from build123d import *

# Parameters (mm, degrees)
SKETCH_1_R         = 3.4
EXTRUDE_1267_DEPTH = 150


with BuildPart() as part:
    # 草圖1 → Extrude 1267 (new body, symmetric)
    with BuildSketch(Plane.XY):
        with BuildLine():
            Line((4.3, 25), (25, 25))
            Line((25, 25), (25, 4.3))
            Line((25, 4.3), (22, 4.3))
            Line((22, 4.3), (22, 6.687301399))
            Line((22, 6.687301399), (14.5, 6.687301399))
            ThreePointArc((14.5, 6.687301399), (10.2, 0), (14.5, -6.687301399))
            Line((14.5, -6.687301399), (22, -6.687301399))
            Line((22, -6.687301399), (22, -4.3))
            Line((22, -4.3), (25, -4.3))
            Line((25, -4.3), (25, -25))
            Line((25, -25), (4.3, -25))
            Line((4.3, -25), (4.3, -22))
            Line((4.3, -22), (6.687301399, -22))
            Line((6.687301399, -22), (6.687301399, -14.5))
            ThreePointArc((6.687301399, -14.5), (0, -10.2), (-6.687301399, -14.5))
            Line((-6.687301399, -14.5), (-6.687301399, -22))
            Line((-6.687301399, -22), (-4.3, -22))
            Line((-4.3, -22), (-4.3, -25))
            Line((-4.3, -25), (-25, -25))
            Line((-25, -25), (-25, -4.3))
            Line((-25, -4.3), (-22, -4.3))
            Line((-22, -4.3), (-22, -6.687301399))
            Line((-22, -6.687301399), (-14.5, -6.687301399))
            ThreePointArc((-14.5, -6.687301399), (-10.2, 0), (-14.5, 6.687301399))
            Line((-14.5, 6.687301399), (-22, 6.687301399))
            Line((-22, 6.687301399), (-22, 4.3))
            Line((-22, 4.3), (-25, 4.3))
            Line((-25, 4.3), (-25, 25))
            Line((-25, 25), (-4.3, 25))
            Line((-4.3, 25), (-4.3, 22))
            Line((-4.3, 22), (-6.687301399, 22))
            Line((-6.687301399, 22), (-6.687301399, 14.5))
            ThreePointArc((-6.687301399, 14.5), (0, 10.2), (6.687301399, 14.5))
            Line((6.687301399, 14.5), (6.687301399, 22))
            Line((6.687301399, 22), (4.3, 22))
            Line((4.3, 22), (4.3, 25))
        make_face()
        with Locations((12.75, 12.75)):
            Circle(SKETCH_1_R, mode=Mode.SUBTRACT)
        with Locations((12.75, -12.75)):
            Circle(SKETCH_1_R, mode=Mode.SUBTRACT)
        with Locations((-12.75, -12.75)):
            Circle(SKETCH_1_R, mode=Mode.SUBTRACT)
        with Locations((-12.75, 12.75)):
            Circle(SKETCH_1_R, mode=Mode.SUBTRACT)
        with BuildLine():
            Line((9.35, 23), (23, 23))
            Line((23, 23), (23, 9.35))
            Line((23, 9.35), (16.945235393, 9.35))
            ThreePointArc((16.945235393, 9.35), (16.568376618, 16.568376618), (9.35, 16.945235393))
            Line((9.35, 16.945235393), (9.35, 23))
        make_face(mode=Mode.SUBTRACT)
        with BuildLine():
            Line((9.35, -23), (9.35, -16.945235393))
            ThreePointArc((9.35, -16.945235393), (16.568376618, -16.568376618), (16.945235393, -9.35))
            Line((16.945235393, -9.35), (23, -9.35))
            Line((23, -9.35), (23, -23))
            Line((23, -23), (9.35, -23))
        make_face(mode=Mode.SUBTRACT)
        with BuildLine():
            Line((-9.35, -23), (-23, -23))
            Line((-23, -23), (-23, -9.35))
            Line((-23, -9.35), (-16.945235393, -9.35))
            ThreePointArc((-16.945235393, -9.35), (-16.568376618, -16.568376618), (-9.35, -16.945235393))
            Line((-9.35, -16.945235393), (-9.35, -23))
        make_face(mode=Mode.SUBTRACT)
        with BuildLine():
            Line((-9.35, 23), (-9.35, 16.945235393))
            ThreePointArc((-9.35, 16.945235393), (-16.568376618, 16.568376618), (-16.945235393, 9.35))
            Line((-16.945235393, 9.35), (-23, 9.35))
            Line((-23, 9.35), (-23, 23))
            Line((-23, 23), (-9.35, 23))
        make_face(mode=Mode.SUBTRACT)
        with BuildLine():
            ThreePointArc((11.864845961, 7.423040048), (8.2, 0), (11.864845961, -7.423040048))
            ThreePointArc((11.864845961, -7.423040048), (8.931623382, -8.931623382), (7.423040048, -11.864845961))
            ThreePointArc((7.423040048, -11.864845961), (0, -8.2), (-7.423040048, -11.864845961))
            ThreePointArc((-7.423040048, -11.864845961), (-8.931623382, -8.931623382), (-11.864845961, -7.423040048))
            ThreePointArc((-11.864845961, -7.423040048), (-8.2, 0), (-11.864845961, 7.423040048))
            ThreePointArc((-11.864845961, 7.423040048), (-8.931623382, 8.931623382), (-7.423040048, 11.864845961))
            ThreePointArc((-7.423040048, 11.864845961), (0, 8.2), (7.423040048, 11.864845961))
            ThreePointArc((7.423040048, 11.864845961), (8.931623382, 8.931623382), (11.864845961, 7.423040048))
        make_face(mode=Mode.SUBTRACT)
    extrude(amount=EXTRUDE_1267_DEPTH, both=True)


solid = part.part
Work out the finished part from the listing and answer in its coordinate system (mm). A direction names the side the tool comes from. Coordinates: 2 decimals unless noted, no trailing zeros. Order: outer loops, then holes, each group sorted by start corner. A loop starts at its lowest first (then second) coordinate and runs counter-clockwise, first axis right, second up. Notation, with made-up numbers: (-7.75, 21) - (29.25, 21) arc R15 ccw to (29.25, 46) - close; hole circle Ø4 at (80, 18.25). An arc over 180 degrees is marked (long way). Put each result on its own line as item: value. Start each with the question number.
1) Find section A-A (x = -0.5). Give the vertices of the cut face in (y, z), plus the area to 3 significant figures.
2) For a pull along Y with two mould halves and no side action, classify faces 3 (the flat face through (15, 25, 2)), 4 (the flat face through (-15, -25, 2)), 5 (the flat face through (-9.35, 20, 2)), 6 (the cylindrical face through (12.01, -16.07, -2.1)) as released by +Y, released by -Y, zero draft, split by the parting line, or undercut.
3) Flat-ended cylindrical pins translate along their axes: pin 1 (3 mm diameter, centred on y = -1.5, z = 65, fed in from +X); pin 2 (4 mm diameter, centred on x = 12.75, y = 12.75, fed in from +Z); pin 3 (4 mm diameter, centred on x = 15.5, y = -19.5, fed in from -Z). Find the tip coordinate at first contact, or state that the pin passes through.
4) Find the intervals of material crossed by line 1 (Y direction, x = 18.5, z = 101); line 2 (Y direction, x = -15, z = -81); line 3 (X direction, y = -12, z = 12), in increasing order. Write a range as from..to.
5) Find section B-B (z = -10.5). State how many separate pieces and enclosed holes the cut face has, plus the area to 3 significant figures.
6) For faces 1 (the flat face through (18, -6.687, 2)), 2 (the flat face through (0, -9, 150)), determine the directions among +Z, -Z, +X, -X, +Y, -Y from which every point of the face is accessible in a straight line to the end or side of a thin tool.
Results list:
1. outline: (-10.22, -150) - (-8.21, -150) - (-8.21, 150) - (-10.22, 150) - close; (8.21, -150) - (10.22, -150) - (10.22, 150) - (8.21, 150) - close
1. area: 1,200 mm^2
2. face 3: released by +Y
2. face 4: released by -Y
2. face 5: undercut
2. face 6: undercut
3. pin 1: stops at x = 10.84
3. pin 2: passes through
3. pin 3: stops at z = -150
4. line 1: y = -25..-23, -9.35..-6.69, 6.69..9.35, 23..25
4. line 2: y = -25..-23, -17.66..-15.3, -10.2..-6.69, 6.69..10.2, 15.3..17.66, 23..25
4. line 3: x = -25..-23, -18.1..-16.07, -9.43..-4.82, 4.82..9.43, 16.07..18.1, 23..25
5. separate pieces: 1
5. enclosed holes: 9
5. area: 859 mm^2
6. face 1: +Z, -Z
6. face 2: +Z, +X, -X, +Y, -Y
